Part model, mm, in its own coordinate system. A direction names the side the tool comes from. Coordinates: 2 decimals unless noted, no trailing zeros. Order: outer loops, then holes, each group sorted by start corner. A loop starts at its lowest first (then second) coordinate and runs counter-clockwise, first axis right, second up. Notation, with made-up numbers: (60.5, -9) - (93.5, -9) arc R13 cw to (93.5, 4) - close; hole circle Ø5 at (62.25, 39.25). An arc over 180 degrees is marked (long way). Use a Markdown table: item, result. Add a question column.
1) Saw through at D-D on x = -27. List the corners of the cut face in (y, z).
2) Saw through at C-C on z = 0.9. Count the separate pieces of the cut face and the enclosed holes in it, then the cut area to 3 significant figures.
3) Tool access for faces 1 (the face through (-4.05, -11.48, 3.97)), 2 (the face through (-4, -4, 3)), 3 (the face through (2, 26, 2)): list every direction of +Z, -Z, +X, -X, +Y, -Y with a clear straight run to the whole face (end or side of a thin tool).
4) Saw through at A-A on x = 0. List the corners of the cut face in (y, z).
5) Wall check: L1, parallel to Y at x = -21.5, z = 3.55; L2, parallel to Z at x = 5.5, y = 11; L3, parallel to Y at x = 27, z = 3. Give the ranges that are in metal, low to high. Write a range as [from, to].
6) Drop flat-ended pins along their axis: P1, Ø3, axis at x = 8, z = 2, coming from the -Y side; P2, Ø1, axis at x = -0.5, z = 1.5, coming from the -Y side; P3, Ø4, axis at x = 11.73, y = -4.86, coming from the -Z side; P4, Ø1.9, axis at x = 19.09, y = 19.09, coming from the +Z side. Give the stop position or say it passes through.
7) Two-plate mould, pull along Y, no slides. Class faces 4 (the face through (6, -6, 0)), 5 (the face through (-13.766, 4.017, 0.986)), 6 (the face through (-4.036, 30.736, 2.958)), 7 (the face through (13.35, -3.37, 0.99)): +Y half, -Y half, draft (parallel to the pull), parting line (faces both ways), or undercut.
```python
from build123d import *

# Parameters (mm, degrees)
SKETCH1_R           = 31
SKETCH1_R_2         = 4.5
SKETCH1_R_3         = 0.85
SKETCH1_R_4         = 1.55
BOSS_EXTRUDE2_DEPTH = 6
SKETCH5_R           = 8.2
CUT_EXTRUDE3_DEPTH  = 3
SKETCH6_R           = 3.5
CUT_EXTRUDE4_DEPTH  = 4
SKETCH7_R           = 2.2
CUT_EXTRUDE5_DEPTH  = 2


with BuildPart() as part:
    # Sketch1 → Boss-Extrude2 (new body)
    with BuildSketch(Plane.XY):
        Circle(SKETCH1_R)
        Circle(SKETCH1_R_2, mode=Mode.SUBTRACT)
        with Locations((4.860079591, 11.733270063)):
            Circle(SKETCH1_R_3, mode=Mode.SUBTRACT)
        with Locations((11.733270063, -4.860079591)):
            Circle(SKETCH1_R_3, mode=Mode.SUBTRACT)
        with Locations((-4.860079591, -11.733270063)):
            Circle(SKETCH1_R_3, mode=Mode.SUBTRACT)
        with Locations((-11.733270063, 4.860079591)):
            Circle(SKETCH1_R_3, mode=Mode.SUBTRACT)
        with Locations((-27, 0)):
            Circle(SKETCH1_R_4, mode=Mode.SUBTRACT)
        with Locations((-19.091883092, 19.091883092)):
            Circle(SKETCH1_R_4, mode=Mode.SUBTRACT)
        with Locations((0, 27)):
            Circle(SKETCH1_R_4, mode=Mode.SUBTRACT)
        with Locations((19.091883092, 19.091883092)):
            Circle(SKETCH1_R_4, mode=Mode.SUBTRACT)
        with Locations((27, 0)):
            Circle(SKETCH1_R_4, mode=Mode.SUBTRACT)
        with Locations((19.091883092, -19.091883092)):
            Circle(SKETCH1_R_4, mode=Mode.SUBTRACT)
        with Locations((0, -27)):
            Circle(SKETCH1_R_4, mode=Mode.SUBTRACT)
        with Locations((-19.091883092, -19.091883092)):
            Circle(SKETCH1_R_4, mode=Mode.SUBTRACT)
    extrude(amount=BOSS_EXTRUDE2_DEPTH)

    # Sketch5 → Cut-Extrude3 (cut)
    with BuildSketch(Plane(origin=(0, 0, 0), x_dir=(-1, 0, 0), z_dir=(0, 0, -1))):
        Circle(SKETCH5_R)
    extrude(amount=-CUT_EXTRUDE3_DEPTH, mode=Mode.SUBTRACT)

    # Sketch6 → Cut-Extrude4 (cut)
    with BuildSketch(Plane.XY.offset(6)):
        with Locations((0, 27)):
            Circle(SKETCH6_R)
        with Locations((19.091883092, 19.091883092)):
            Circle(SKETCH6_R)
        with Locations((27, 0)):
            Circle(SKETCH6_R)
        with Locations((19.091883092, -19.091883092)):
            Circle(SKETCH6_R)
        with Locations((0, -27)):
            Circle(SKETCH6_R)
        with Locations((-19.091883092, -19.091883092)):
            Circle(SKETCH6_R)
        with Locations((-27, 0)):
            Circle(SKETCH6_R)
        with Locations((-19.091883092, 19.091883092)):
            Circle(SKETCH6_R)
    extrude(amount=-CUT_EXTRUDE4_DEPTH, mode=Mode.SUBTRACT)

    # Sketch7 → Cut-Extrude5 (cut)
    with BuildSketch(Plane(origin=(0, 0, 0), x_dir=(-1, 0, 0), z_dir=(0, 0, -1))):
        with Locations((-4.860079591, 11.733270063)):
            Circle(SKETCH7_R)
        with Locations((11.733270063, 4.860079591)):
            Circle(SKETCH7_R)
        with Locations((4.860079591, -11.733270063)):
            Circle(SKETCH7_R)
        with Locations((-11.733270063, -4.860079591)):
            Circle(SKETCH7_R)
    extrude(amount=-CUT_EXTRUDE5_DEPTH, mode=Mode.SUBTRACT)


solid = part.part
```
Results are:
| question | item | result |
|---|---|---|
| 1 | outline | (-15.23, 0) - (-1.55, 0) - (-1.55, 2) - (-3.5, 2) - (-3.5, 6) - (-15.23, 6) - close; (1.55, 0) - (15.23, 0) - (15.23, 6) - (3.5, 6) - (3.5, 2) - (1.55, 2) - close |
| 2 | separate pieces | 1 |
| 2 | enclosed holes | 13 |
| 2 | area | 2,690 mm2 |
| 3 | face 1 | +Z, -Z |
| 3 | face 2 | -Z |
| 3 | face 3 | +Z |
| 4 | outline | (-31, 0) - (-28.55, 0) - (-28.55, 2) - (-30.5, 2) - (-30.5, 6) - (-31, 6) - close; (-25.45, 0) - (-8.2, 0) - (-8.2, 3) - (-4.5, 3) - (-4.5, 6) - (-23.5, 6) - (-23.5, 2) - (-25.45, 2) - close; (4.5, 3) - (8.2, 3) - (8.2, 0) - (25.45, 0) - (25.45, 2) - (23.5, 2) - (23.5, 6) - (4.5, 6) - close; (28.55, 0) - (31, 0) - (31, 6) - (30.5, 6) - (30.5, 2) - (28.55, 2) - close |
| 5 | L1 | [-22.33, -21.63], [-16.55, 16.55], [21.63, 22.33] |
| 5 | L2 | [2, 6] |
| 5 | L3 | [-15.23, -3.5], [3.5, 15.23] |
| 6 | P1 | y = -30.31 |
| 6 | P2 | y = -31 |
| 6 | P3 | z = 2 |
| 6 | P4 | through |
| 7 | face 4 | draft |
| 7 | face 5 | undercut |
| 7 | face 6 | parting line |
| 7 | face 7 | undercut |
